```python
from build123d import *

# Parameters (mm, degrees)
CHASIS_W                = 533.4
CHASIS_H                = 279.4
BOSS_EXTRUDE1_DEPTH     = 152.4
SKETCH3_W               = 63.5
SKETCH3_H               = 50.8
MIRROR2_COPY_1_SKETCH_W = 63.5
MIRROR2_COPY_1_SKETCH_H = 50.8
SKETCH4_W               = 101.6
SKETCH4_H               = 12.7
CUT_EXTRUDE1_DEPTH      = 241.3
BOSS_EXTRUDE2_DEPTH     = 101.6


with BuildPart() as part:
    # Chasis → Boss-Extrude1 (new body)
    with BuildSketch(Plane(origin=(0, 0, 0), x_dir=(1, 0, 0), z_dir=(0, 1, 0))):
        Rectangle(CHASIS_W, CHASIS_H)
    extrude(amount=BOSS_EXTRUDE1_DEPTH)

    # Sketch3 → Revolve2 (revolve)
    with BuildSketch(Plane(origin=(0, 38.1, 0), x_dir=(-1, 0, 0), z_dir=(0, -1, 0))):
        with Locations((215.9, -95.25)):
            Rectangle(SKETCH3_W, SKETCH3_H)
    revolve2 = revolve(axis=Axis((-184.15, 38.1, 69.85), (0, 0, 1)))

    # Mirror1: Revolve2 across plane
    add(revolve2.mirror(Plane.XY))

    # Mirror2: Revolve2 across plane
    add(revolve2.mirror(Plane(origin=(0, 0, 0), x_dir=(0, 0, 1), z_dir=(1, 0, 0))))

    # Mirror2 copy 1 sketch → Mirror2 copy 1 (revolve)
    with BuildSketch(Plane.XZ.offset(-38.1)):
        with Locations((215.9, -95.25)):
            Rectangle(MIRROR2_COPY_1_SKETCH_W, MIRROR2_COPY_1_SKETCH_H)
    revolve(axis=Axis((184.15, 38.1, -69.85), (0, 0, -1)))

    # Sketch4 → Cut-Extrude1 (cut)
    with BuildSketch(Plane.ZY.offset(266.7)):
        with Locations((0, 44.45)):
            Rectangle(SKETCH4_W, SKETCH4_H)
    extrude(amount=-CUT_EXTRUDE1_DEPTH, mode=Mode.SUBTRACT)

    # Sketch7 → Boss-Extrude2 (add)
    with BuildSketch(Plane.XY.offset(-50.8)):
        Polygon((-266.7, 38.1), (-529.359422098, -25.4), (-515.991575795, -25.4), (-266.7, 33.027558643), align=None)
    extrude(amount=BOSS_EXTRUDE2_DEPTH)


solid = part.part
```
Work out the finished part from the listing and answer in its coordinate system (mm). A direction names the side the tool comes from. Round coordinates to 2 decimals unless told otherwise and drop trailing zeros. Loops run counter-clockwise (first coordinate to the right, second up) from the corner with the lowest first, then second, coordinate; pieces in that order, holes last.
(1) For faces 4 (the flat face through (-185, -10, 120.65)), 5 (the flat face through (-185, -10, 69.85)), 6 (the flat face through (185, -10, -120.65)), determine the directions among +Z, -Z, +X, -X, +Y, -Y from which every point of the face is accessible in a straight line to the end or side of a thin tool.
Computed values:
face 4: +Z, +X, -X, -Y
face 5: +X, -X, -Y
face 6: -Z, +X, -X, -Y
(2) Each of these flat-tipped pins is pushed along its axis until it touches: P1, Ø2, axis at x = -414, z = -26, coming from the +Y side; P2, Ø7.5, axis at x = -203.5, y = -10.5, coming from the -Z side; P3, Ø7.5, axis at x = 184, y = -13.5, coming from the +Z side. Where does it stop, or does it pass through?
Computed values:
P1: stops at y = 2.73
P2: stops at z = -120.65
P3: stops at z = 120.65
(3) The part is cut by section B-B, the plane x = -35.5. Give the vertices of the cut face in (y, z), and give its area (3 significant figures).
Computed values:
outline: (0, -139.7) - (152.4, -139.7) - (152.4, 139.7) - (0, 139.7) - close; hole (38.1, -50.8) - (50.8, -50.8) - (50.8, 50.8) - (38.1, 50.8) - close
area: 41,300 mm2
(4) The mould has two halves that part along X. Classify faces 1 (the flat face through (-396.191, 6.794, -0.711)), 2 (the flat face through (-4, 0, -2)), 3 (the flat face through (-369, 11, 50.8)): pulls with the +X half, pulls with the -X half, needs draft (parallel to the pull), parting line crosses it, or undercut.
Computed values:
face 1: pulls with the -X half
face 2: undercut
face 3: needs draft
(5) Find the intervals of material crossed by L1, parallel to Z at x = -247, y = 43.5; L2, parallel to X at y = 135, z = 3; L3, parallel to Y at x = -75.5, z = 4.5, in increasing order.
Computed values:
L1: z = -139.7 to -50.8, 50.8 to 139.7
L2: x = -266.7 to 266.7
L3: y = 0 to 38.1, 50.8 to 152.4
(6) The part is cut by section C-C, the plane y = -9.5. Give the vertices of the cut face in (x, z).
Computed values:
outline: (-463.59, -50.8) - (-448.15, -50.8) - (-448.15, 50.8) - (-463.59, 50.8) - close; (-226.18, -120.65) - (-142.12, -120.65) - (-142.12, -69.85) - (-226.18, -69.85) - close; (-226.18, 69.85) - (-142.12, 69.85) - (-142.12, 120.65) - (-226.18, 120.65) - close; (142.12, -120.65) - (226.18, -120.65) - (226.18, -69.85) - (142.12, -69.85) - close; (142.12, 69.85) - (226.18, 69.85) - (226.18, 120.65) - (142.12, 120.65) - close
(7) The part is cut by section A-A, the plane z = 98.5. Give the vertices of the cut face in (x, y), and give its area (3 significant figures).
Computed values:
outline: (-266.7, 0) - (-234.95, 0) arc R63.5 ccw to (-133.35, 0) - (133.35, 0) arc R63.5 ccw to (234.95, 0) - (266.7, 0) - (266.7, 152.4) - (-266.7, 152.4) - close
area: 84,900 mm2
(8) The part is cut by section D-D, the plane x = 174. Give the vertices of the cut face in (y, z), and give its area (3 significant figures).
Computed values:
outline: (-24.58, -120.65) - (0, -120.65) - (0, -139.7) - (152.4, -139.7) - (152.4, 139.7) - (0, 139.7) - (0, 120.65) - (-24.58, 120.65) - (-24.58, 69.85) - (0, 69.85) - (0, -69.85) - (-24.58, -69.85) - close
area: 45,100 mm2
